For this review, take the finished solid that the model builds, in its own axes (mm). Face numbers are marked on the shaded views. Coordinates: 2 decimals unless noted, no trailing zeros. Order: outer loops, then holes, each group sorted by start corner. A loop starts at its lowest first (then second) coordinate and runs counter-clockwise, first axis right, second up. Notation, with made-up numbers: (-25, 6.25) - (3, 6.25) arc R30 cw to (3, 32.25) - close; hole circle Ø7 at (32.5, 10). An arc over 180 degrees is marked (long way). One line per item, written item: value. Start each with the question number.
(1) Consider section C-C on z = 1.5. Write out the cut boundary in (x, y).
(2) Consider section D-D on y = -7. Write out the cut boundary in (x, z).
(3) Consider section A-A on x = 22.5. Write out the cut boundary in (y, z).
(4) To check wall thickness, follow line 1 along Y through (x, z) = (22.5, 2.6); line 2 along Y through (x, z) = (17.25, 0.2); line 3 along X through (y, z) = (-51.5, 3.3). State the ranges of each line that lie inside material, in increasing order.
(5) Mouldability with a two-part tool opening along X and no side actions: class the marked faces 1 and 2 as released by +X, released by -X, zero draft, split by the parting line, or undercut.
(6) Consider section B-B on y = -56. Write out the cut boundary in (x, z), then the cut area to 3 significant figures.
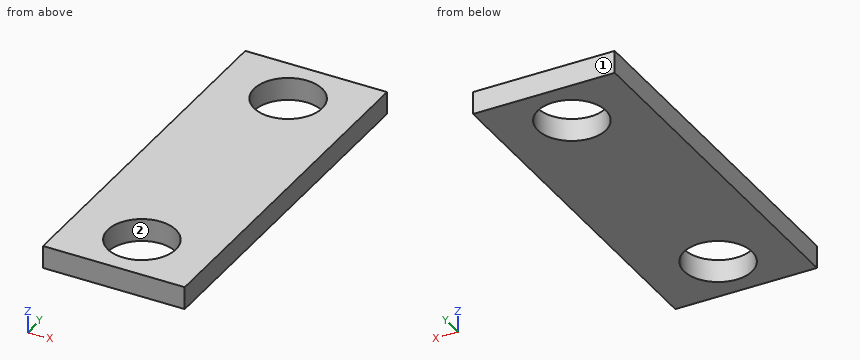
Autodesk Inventor part; units mm, degrees
ref_plane "YZ Plane" through (0, 0, 0) normal (1, 0, 0) x (0, 1, 0)
ref_plane "XZ Plane" through (0, 0, 0) normal (0, 1, 0) x (-1, 0, 0)
ref_plane "XY Plane" through (0, 0, 0) normal (0, 0, 1) x (1, 0, 0)
sketch "Sketch1" plane through (0, 0, 0) normal (0, 0, 1) x (1, 0, 0)
  line L0 (0, 0) -> (45, 0)
  line L1 (45, 0) -> (45, -65)
  line L2 (45, -65) -> (0, -65)
  line L3 (0, -65) -> (0, 0)
  line L4 (45, 15.0081) -> (45, -81.3497) construction
  line L5 (22.5, 15.0081) -> (22.5, -81.3497) construction
  line L6 (80.9794, 0) -> (-24.1636, 0) construction
  line L7 (80.9794, -9) -> (-24.1636, -9) construction
  circle A0 centre (22.5, -9) radius 6
  line L8 (91.2527, -65) -> (-31.7655, -65) construction
  line L9 (91.2527, -56) -> (-31.7655, -56) construction
  circle A1 centre (22.5, -56) radius 6
  line L10 (0, 6.8812) -> (0, -100.7793) construction
  line L11 (10, 6.8812) -> (10, -100.7793)
  line L12 (35, 15.0081) -> (35, -81.3497)
  point P0 (35, -65)
  point P1 (35, 0)
  point P2 (10, 0)
  point P3 (10, -65)
  dimension "d0" = 45
  dimension "d1" = 65
  dimension "d2" = 22.5
  dimension "d3" = 9
  dimension "d4" = 12
  dimension "d5" = 9
  dimension "d6" = 12
  dimension "d9" = 10
  dimension "d10" = 10
extrude "Extrusion2" add sketch "Sketch1" along normal blind 4 contours L0 L12 L2 L11
properties part number "Hook-Extension" material "Steel, Mild"
Geometry check:
1. outline: (10, -65) - (35, -65) - (35, 0) - (10, 0) - close; hole circle Ø12 at (22.5, -56); hole circle Ø12 at (22.5, -9)
2. outline: (10, 0) - (16.84, 0) - (16.84, 4) - (10, 4) - close; (28.16, 0) - (35, 0) - (35, 4) - (28.16, 4) - close
3. outline: (-65, 0) - (-62, 0) - (-62, 4) - (-65, 4) - close; (-50, 0) - (-15, 0) - (-15, 4) - (-50, 4) - close; (-3, 0) - (0, 0) - (0, 4) - (-3, 4) - close
4. line 1: y = -65 to -62, -50 to -15, -3 to 0
4. line 2: y = -65 to -58.9, -53.1 to -11.9, -6.1 to 0
4. line 3: x = 10 to 18.53, 26.47 to 35
5. face 1: zero draft
5. face 2: undercut
6. outline: (10, 0) - (16.5, 0) - (16.5, 4) - (10, 4) - close; (28.5, 0) - (35, 0) - (35, 4) - (28.5, 4) - close
6. area: 52.0 mm^2
